from build123d import *

# Parameters (mm, degrees)
SKETCH2_R           = 30
BOSS_EXTRUDE1_DEPTH = 25


with BuildPart() as part:
    # Sketch2 → Boss-Extrude1 (new body)
    with BuildSketch(Plane.XY):
        with BuildLine():
            Line((63, 107.8), (107.8, 107.8))
            Line((107.8, 107.8), (107.8, 63))
            ThreePointArc((107.8, 63), (98.035981505, 35.080114613), (73, 19.330330892))
            Line((73, 19.330330892), (73, -19.330330892))
            ThreePointArc((73, -19.330330892), (98.035981505, -35.080114613), (107.8, -63))
            Line((107.8, -63), (107.8, -107.8))
            Line((107.8, -107.8), (63, -107.8))
            ThreePointArc((63, -107.8), (31.321616203, -94.678383797), (18.2, -63))
            Line((18.2, -63), (18.2, -53))
            ThreePointArc((18.2, -53), (14.685281374, -44.514718626), (6.2, -41))
            Line((6.2, -41), (-6.2, -41))
            ThreePointArc((-6.2, -41), (-14.685281374, -44.514718626), (-18.2, -53))
            Line((-18.2, -53), (-18.2, -63))
            ThreePointArc((-18.2, -63), (-31.321616203, -94.678383797), (-63, -107.8))
            Line((-63, -107.8), (-107.8, -107.8))
            Line((-107.8, -107.8), (-107.8, -63))
            ThreePointArc((-107.8, -63), (-98.035981505, -35.080114613), (-73, -19.330330892))
            Line((-73, -19.330330892), (-73, 19.330330892))
            ThreePointArc((-73, 19.330330892), (-98.035981505, 35.080114613), (-107.8, 63))
            Line((-107.8, 63), (-107.8, 107.8))
            Line((-107.8, 107.8), (-63, 107.8))
            ThreePointArc((-63, 107.8), (-31.321616203, 94.678383797), (-18.2, 63))
            Line((-18.2, 63), (-18.2, 53))
            ThreePointArc((-18.2, 53), (-14.685281374, 44.514718626), (-6.2, 41))
            Line((-6.2, 41), (6.2, 41))
            ThreePointArc((6.2, 41), (14.685281374, 44.514718626), (18.2, 53))
            Line((18.2, 53), (18.2, 63))
            ThreePointArc((18.2, 63), (31.321616203, 94.678383797), (63, 107.8))
        make_face()
        Circle(SKETCH2_R, mode=Mode.SUBTRACT)
        with BuildLine():
            Line((63, 95.5), (95.5, 95.5))
            Line((95.5, 95.5), (95.5, 63))
            ThreePointArc((95.5, 63), (40.019029611, 40.019029611), (63, 95.5))
        make_face(mode=Mode.SUBTRACT)
        with BuildLine():
            Line((95.5, -95.5), (95.5, -63))
            ThreePointArc((95.5, -63), (40.019029611, -40.019029611), (63, -95.5))
            Line((63, -95.5), (95.5, -95.5))
        make_face(mode=Mode.SUBTRACT)
        with BuildLine():
            Line((-63, -95.5), (-95.5, -95.5))
            Line((-95.5, -95.5), (-95.5, -63))
            ThreePointArc((-95.5, -63), (-40.019029611, -40.019029611), (-63, -95.5))
        make_face(mode=Mode.SUBTRACT)
        with BuildLine():
            Line((-95.5, 95.5), (-95.5, 63))
            ThreePointArc((-95.5, 63), (-40.019029611, 40.019029611), (-63, 95.5))
            Line((-63, 95.5), (-95.5, 95.5))
        make_face(mode=Mode.SUBTRACT)
    extrude(amount=BOSS_EXTRUDE1_DEPTH)


solid = part.part
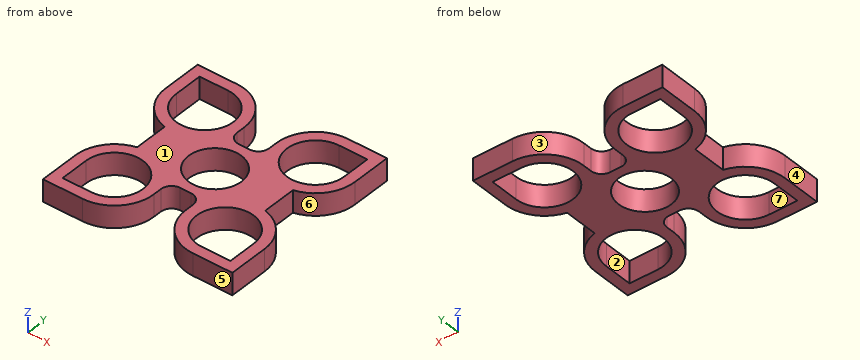
Work out the finished part from the listing and answer in its coordinate system (mm). Face numbers are marked on the shaded views. A direction names the side the tool comes from. Give positions to 0.01 mm unless a question says otherwise; leave off trailing zeros. Loops run counter-clockwise (first coordinate to the right, second up) from the corner with the lowest first, then second, coordinate; pieces in that order, holes last. Notation, with made-up numbers: (41.5, 75) -> (58.5, 75) arc R24 ccw to (58.5, 111) -> close; hole circle Ø9 at (45.5, 79). An arc over 180 degrees is marked (long way). Use a Markdown table: item, result. Add a question column.
1. Determine the mould class of the marked faces 4, 5, 6 and 7 for opening direction Y: released by +Y, released by -Y, zero draft, split by the parting line, or undercut.
2. For the marked faces 1, 2 and 3, determine the directions among +Z, -Z, +X, -X, +Y, -Y from which every point of the face is accessible in a straight line to the end or side of a thin tool.
3. Find the intervals of material crossed by probe 1 along X at (y, z) = (-63, 17.75); probe 2 along Y at (x, z) = (63, 9.25); probe 3 along Y at (x, z) = (-48, 10.5), in increasing order.
4. Section C-C on x = 90.5 is taken. Determine the outline of the cut face in (y, z), and give its area (3 significant figures).
5. Section A-A on x = 0 is taken. Determine the outline of the cut face in (y, z), and give its area (3 significant figures).
6. Section B-B on y = 0 is taken. Determine the outline of the cut face in (x, z).
7. Section D-D on y = 47 is taken. Determine the outline of the cut face in (x, z), and give its area (3 significant figures).
8. Flat-ended cylindrical pins translate along their axes: pin 1 Ø12.5 at (y, z) = (6.5, 16.5) entering from +X; pin 2 Ø1 at (y, z) = (16, 9.5) entering from -X; pin 3 Ø10 at (x, y) = (-38, 60) entering from -Z; pin 4 Ø10 at (y, z) = (53.5, 19) entering from -X. Find the tip coordinate at first contact, or state that the pin passes through.
Results below:
| question | item | result |
|---|---|---|
| 1 | face 4 | zero draft |
| 1 | face 5 | released by -Y |
| 1 | face 6 | undercut |
| 1 | face 7 | undercut |
| 2 | face 1 | +Z, +X, -X, +Y, -Y |
| 2 | face 2 | +Z, -Z |
| 2 | face 3 | +Z, -Z, +Y |
| 3 | probe 1 | x = -107.8 to -95.5, -30.5 to -18.2, 18.2 to 30.5, 95.5 to 107.8 |
| 3 | probe 2 | y = -107.8 to -95.5, -30.5 to 30.5, 95.5 to 107.8 |
| 3 | probe 3 | y = -105.21 to -91.83, -34.17 to 34.17, 91.83 to 105.21 |
| 4 | outline | (-107.8, 0) -> (-95.5, 0) -> (-95.5, 25) -> (-107.8, 25) -> close; (-45.68, 0) -> (-27.63, 0) -> (-27.63, 25) -> (-45.68, 25) -> close; (27.63, 0) -> (45.68, 0) -> (45.68, 25) -> (27.63, 25) -> close; (95.5, 0) -> (107.8, 0) -> (107.8, 25) -> (95.5, 25) -> close |
| 4 | area | 1,520 mm^2 |
| 5 | outline | (-41, 0) -> (-30, 0) -> (-30, 25) -> (-41, 25) -> close; (30, 0) -> (41, 0) -> (41, 25) -> (30, 25) -> close |
| 5 | area | 550 mm^2 |
| 6 | outline | (-73, 0) -> (-30, 0) -> (-30, 25) -> (-73, 25) -> close; (30, 0) -> (73, 0) -> (73, 25) -> (30, 25) -> close |
| 7 | outline | (-104.85, 0) -> (-91.29, 0) -> (-91.29, 25) -> (-104.85, 25) -> close; (-34.71, 0) -> (-16.59, 0) -> (-16.59, 25) -> (-34.71, 25) -> close; (16.59, 0) -> (34.71, 0) -> (34.71, 25) -> (16.59, 25) -> close; (91.29, 0) -> (104.85, 0) -> (104.85, 25) -> (91.29, 25) -> close |
| 7 | area | 1,580 mm^2 |
| 8 | pin 1 | stops at x = 73 |
| 8 | pin 2 | stops at x = -73 |
| 8 | pin 3 | passes through |
| 8 | pin 4 | stops at x = -107.57 |
